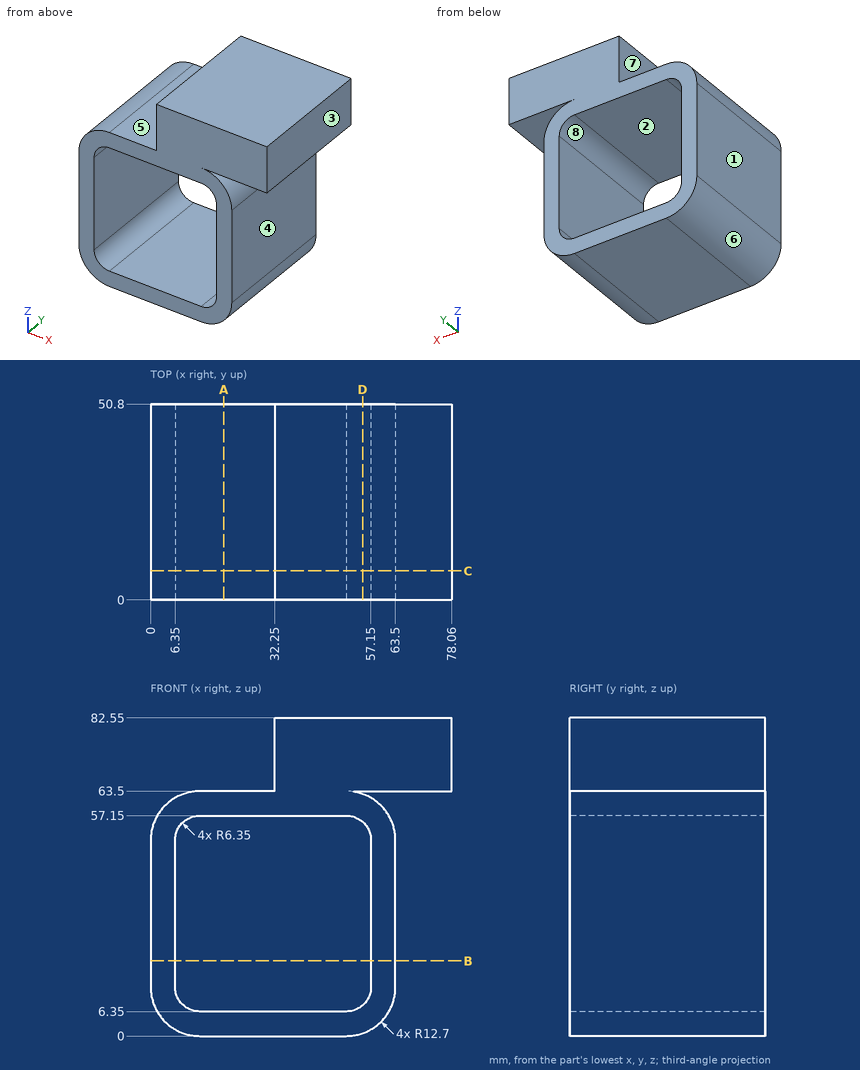
Geometry check sheet. Reference: drawing and pictorial views, mm from the part's lowest x, y, z. A direction names the side the tool comes from. Round coordinates to 2 decimals unless told otherwise and drop trailing zeros. Loops run counter-clockwise (first coordinate to the right, second up) from the corner with the lowest first, then second, coordinate; pieces in that order, holes last.
1. Gauge pin test, flat ends, axial feed: pin 1 Ø1.5 at (x, y) = (65, 31) entering from -Z; pin 2 Ø8 at (x, y) = (65.5, 25.5) entering from -Z; pin 3 Ø11.5 at (y, z) = (19, 30.5) entering from +X. Record the tip position at first contact, or that the pin passes through.
2. Sectioned sample at C-C on y = 7.5. Record the boundary of the cut face in (x, z), and give its area (3 significant figures).
3. Set-up check for the marked faces 1, 2, 3, 4 and 5: record each of +Z, -Z, +X, -X, +Y, -Y from which the full face is reachable in a straight line by a thin tool's end or side.
4. Mould release check, pull along Z, two halves, no side actions. Record for the marked faces 6, 7 and 8: released by +Z, released by -Z, zero draft, split by the parting line, or undercut.
5. Sectioned sample at B-B on z = 19.5. Record the boundary of the cut face in (x, y).
6. Sectioned sample at D-D on x = 55. Record the boundary of the cut face in (y, z).
7. Sectioned sample at A-A on x = 19. Record the boundary of the cut face in (y, z).
8. Scan lines: probe 1 along Z at (x, y) = (30.5, 47); probe 2 along Z at (x, y) = (50, 13). Record each from-to range of solid material in increasing order.
Recorded:
1. pin 1: stops at z = 63.5
1. pin 2: stops at z = 5.86
1. pin 3: stops at x = 63.5
2. outline: (0, 12.7) arc R12.7 ccw to (12.7, 0) - (50.8, 0) arc R12.7 ccw to (63.5, 12.7) - (63.5, 50.8) arc R12.7 ccw to (50.8, 63.5) - (78.06, 63.5) - (78.06, 82.55) - (32.25, 82.55) - (32.25, 63.5) - (12.7, 63.5) arc R12.7 ccw to (0, 50.8) - close; hole (6.35, 12.7) arc R6.35 ccw to (12.7, 6.35) - (50.8, 6.35) arc R6.35 ccw to (57.15, 12.7) - (57.15, 50.8) arc R6.35 ccw to (50.8, 57.15) - (12.7, 57.15) arc R6.35 ccw to (6.35, 50.8) - close
2. area: 2,220 mm2
3. face 1: +Z, -Z, -X, +Y, -Y
3. face 2: +Y, -Y
3. face 3: +Z, -Z, +X, +Y, -Y
3. face 4: -Z, +X, +Y, -Y
3. face 5: +Z, -X, +Y, -Y
4. face 6: released by -Z
4. face 7: zero draft
4. face 8: undercut
5. outline: (0, 0) - (6.35, 0) - (6.35, 50.8) - (0, 50.8) - close; (57.15, 0) - (63.5, 0) - (63.5, 50.8) - (57.15, 50.8) - close
6. outline: (0, 0.71) - (50.8, 0.71) - (50.8, 7.94) - (0, 7.94) - close; (0, 55.56) - (50.8, 55.56) - (50.8, 62.79) - (0, 62.79) - close; (0, 63.5) - (50.8, 63.5) - (50.8, 82.55) - (0, 82.55) - close
7. outline: (0, 0) - (50.8, 0) - (50.8, 6.35) - (0, 6.35) - close; (0, 57.15) - (50.8, 57.15) - (50.8, 63.5) - (0, 63.5) - close
8. probe 1: z = 0 to 6.35, 57.15 to 63.5
8. probe 2: z = 0 to 6.35, 57.15 to 82.55
